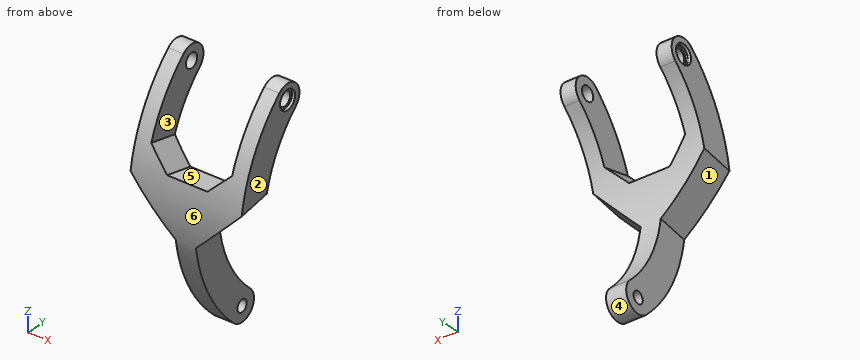
from build123d import *

# Parameters (mm, degrees)
SKETCH_1_R               = 1.175
SKETCH_1_R_2             = 1.425
EXTRUDE_1_DEPTH          = 11
CUT_EXTRUDE_1_DEPTH      = 8
CUT_EXTRUDE_1_DEPTH_BACK = 8
SKETCH_1_6_R             = 1.425
SKETCH_4_R               = 1.175
CUT_EXTRUDE_3_DEPTH      = 9
CUT_EXTRUDE_START        = -0.6
SKETCH_6_R               = 1.9
CUT_EXTRUDE_5_DEPTH      = 35.929603411
SKETCH_3_R               = 1.85
CUT_EXTRUDE_2_DEPTH      = 1
CHAMFER_2_SIZE           = 10
CHAMFER_3_SIZE           = 4


with BuildPart() as part:
    # 草图1 → 凸台-拉伸1 (new, symmetric)
    with BuildSketch(Plane(origin=(0, 0, 0), x_dir=(0, 0, -1), z_dir=(1, 0, 0))):
        with BuildLine():
            ThreePointArc((-22.696428571, -2.043453335), (0, -11.927768877), (22.696428571, -2.043453335))
            ThreePointArc((22.696428571, -2.043453335), (22.543453335, 2.196428571), (18.303571429, 2.043453335))
            ThreePointArc((18.303571429, 2.043453335), (0, -5.927768877), (-18.303571429, 2.043453335))
            ThreePointArc((-18.303571429, 2.043453335), (-22.543453335, 2.196428571), (-22.696428571, -2.043453335))
        make_face()
        with Locations((20.5, 0)):
            Circle(SKETCH_1_R, mode=Mode.SUBTRACT)
        with Locations((-20.5, 0)):
            Circle(SKETCH_1_R_2, mode=Mode.SUBTRACT)
    extrude(amount=EXTRUDE_1_DEPTH, both=True)

    # 草图1<6> → 切除-拉伸1 (cut, two sides: drawn at the far end of the back side and taken through both)
    with BuildSketch(Plane(origin=(0, 0, 0), x_dir=(0, 0, -1), z_dir=(1, 0, 0)).offset(-CUT_EXTRUDE_1_DEPTH_BACK)):
        with BuildLine():
            ThreePointArc((-22.696428571, -2.043453335), (-15.296359873, -7.89110277), (-6.48036682, -11.242861585))
            Line((-6.48036682, -11.242861585), (-5.226102274, -5.375424287))
            ThreePointArc((-5.226102274, -5.375424287), (-12.335774091, -2.672392985), (-18.303571429, 2.043453335))
            ThreePointArc((-18.303571429, 2.043453335), (-22.543453335, 2.196428571), (-22.696428571, -2.043453335))
        make_face()
        with Locations((-20.5, 0)):
            Circle(SKETCH_1_6_R, mode=Mode.SUBTRACT)
    extrude(amount=CUT_EXTRUDE_1_DEPTH + CUT_EXTRUDE_1_DEPTH_BACK, mode=Mode.SUBTRACT)

    # 草图4 → 切除-拉伸3 (cut)
    with BuildSketch(Plane(origin=(11, 0, 0), x_dir=(0, 0, -1), z_dir=(1, 0, 0))):
        with BuildLine():
            ThreePointArc((18.303571429, 2.043453335), (11.941686142, -2.891287085), (4.341204442, -5.547962703))
            Line((4.341204442, -5.547962703), (5.383093508, -11.456809221))
            ThreePointArc((5.383093508, -11.456809221), (14.807690816, -8.162531455), (22.696428571, -2.043453335))
            ThreePointArc((22.696428571, -2.043453335), (23.487928503, 0.268855462), (22.296358841, 2.402726558))
            ThreePointArc((22.296358841, 2.402726558), (20.231144538, 2.987928503), (18.303571429, 2.043453335))
        make_face()
        with Locations((20.5, 0)):
            Circle(SKETCH_4_R, mode=Mode.SUBTRACT)
    cut_extrude_3 = extrude(amount=-CUT_EXTRUDE_3_DEPTH, mode=Mode.SUBTRACT)

    # 草图6 → 切除-拉伸5 (cut)
    with BuildSketch(Plane(origin=(11, 0, 0), x_dir=(0, 0, -1), z_dir=(1, 0, 0)).offset(CUT_EXTRUDE_START)):
        with Locations(Location((-20.5, 0, 0), (0, 0, 180))):
            Circle(SKETCH_6_R)
    cut_extrude_5 = extrude(amount=CUT_EXTRUDE_5_DEPTH, mode=Mode.SUBTRACT)

    # 镜向3: 切除-拉伸3, 切除-拉伸5 across plane
    add(cut_extrude_3.mirror(Plane(origin=(0, 0, 0), x_dir=(0, 0, 1), z_dir=(1, 0, 0))), mode=Mode.SUBTRACT)
    add(cut_extrude_5.mirror(Plane(origin=(0, 0, 0), x_dir=(0, 0, 1), z_dir=(1, 0, 0))), mode=Mode.SUBTRACT)

    # 草图3 → 切除-拉伸2 (cut)
    with BuildSketch(Plane.ZY.offset(11)):
        with Locations((20.5, 0)):
            Circle(SKETCH_3_R)
    extrude(amount=-CUT_EXTRUDE_2_DEPTH, mode=Mode.SUBTRACT)

    # 倒角2
    # the kernel refuses this chamfer: 10 mm, written as the material it adds along each edge
    # the kernel refuses this chamfer: 10 mm, written as the material it takes off along each edge
    with BuildSketch(Plane(origin=(-11, 19.778170746, 0.124476202), x_dir=(-0.027495876610586313, -0.1735825242275637, 0.9844354138551714), z_dir=(0, -0.9848077530122094, -0.17364817766692373))) as chamfer_2_2_piece_1_section:
        Polygon((CHAMFER_2_SIZE * 0.999621916911, -CHAMFER_2_SIZE * 0.0274958766106), (-CHAMFER_2_SIZE * 0.0274958766106, -CHAMFER_2_SIZE * 0.999621916911), (0, 0), align=None)
    chamfer_2_2_piece_1 = extrude(amount=57.433659759, mode=Mode.PRIVATE)
    chamfer_2_2_piece_1 = split(chamfer_2_2_piece_1, bisect_by=Plane(origin=(-2, -8.783186583, -1.465639678), z_dir=(-1, 0, 0)), keep=Keep.TOP, mode=Mode.PRIVATE)
    add(chamfer_2_2_piece_1, mode=Mode.SUBTRACT)
    with BuildSketch(Plane(origin=(11, 19.778170746, 0.124476202), x_dir=(-0.9996219169112968, 0.004774608866782908, -0.027078152461972493), z_dir=(0, -0.9848077530122094, -0.17364817766692373))) as chamfer_2_2_piece_2_section:
        Polygon((CHAMFER_2_SIZE * 0.999621916911, -CHAMFER_2_SIZE * 0.0274958766106), (-CHAMFER_2_SIZE * 0.0274958766106, -CHAMFER_2_SIZE * 0.999621916911), (0, 0), align=None)
    chamfer_2_2_piece_2 = extrude(amount=57.433659759, mode=Mode.PRIVATE)
    chamfer_2_2_piece_2 = split(chamfer_2_2_piece_2, bisect_by=Plane(origin=(2, -8.783186583, -1.465639678), z_dir=(1, 0, 0)), keep=Keep.TOP, mode=Mode.PRIVATE)
    add(chamfer_2_2_piece_2, mode=Mode.SUBTRACT)

    # 倒角3
    chamfer_3_edges = [part.edges().sort_by_distance(p)[0] for p in [
        (8, -8.309142936, 5.853234547),
        (-8, -8.309142936, 5.853234547),
    ]]
    chamfer(chamfer_3_edges, length=CHAMFER_3_SIZE)


solid = part.part
Build history of the part. All positions in model axes, mm. Face numbers are marked on the shaded views. A direction names the side the tool comes from. Give positions to 0.01 mm unless a question says otherwise; leave off trailing zeros. Write each loop counter-clockwise with the first axis right and the second up, starting at its lowest first coordinate (ties: lowest second). Pieces come first, ordered by that corner, then holes. Notation, with made-up numbers: (3, 21) - (60, 21) arc R23 ccw to (60, 50) - close; hole circle Ø11 at (6, 82.25). An arc over 180 degrees is marked (long way). Use one line per item in the form item = value. Start each with the question number.
1. Band-saw the part on D-D on z = 20.5. Write the cut outline in (x, y) (3 decimals).
2. Two-plate mould, pull along X, no slides. Class the marked faces 1, 2, 3 and 4: released by +X, released by -X, zero draft, split by the parting line, or undercut.
3. Band-saw the part on B-B on z = 7.5. Write the cut outline in (x, y), plus the area to 3 significant figures.
4. Band-saw the part on A-A on x = -0.25. Write the cut outline in (y, z) (3 decimals), plus the area to 3 significant figures.
5. 3-axis set-ups, long thin cutter, end or side, ignore diameter. For the marked faces 5 and 6: which of +Z, -Z, +X, -X, +Y, -Y reach the whole face in a straight line?
6. Probe line 1 (X direction, y = -3.25, z = 16); line 2 (Y direction, x = -0.35, z = -20.5) (3 decimals); line 3 (Z direction, x = 0.25, y = 0.75). List the from-to ranges inside material, lowest first. Write a range as [from, to].
7. Drop flat-ended pins along their axis: pin 1 Ø1 at (x, y) = (-8, -4.5) entering from +Z; pin 2 Ø2 at (x, z) = (-2.5, -13.5) entering from +Y; pin 3 Ø1.1 at (y, z) = (1, 21) entering from -X. Give the stop position or say it passes through.
8. Band-saw the part on C-C on y = -2.5. Write the cut outline in (x, z), plus the area to 3 significant figures.
Conclusion:
q1.outline = (-11, -4.182) - (-8, -4.182) - (-8, -1.425) - (-10, -1.425) - (-10, -1.85) - (-10.4, -1.85) - (-10.4, -1.9) - (-11, -1.9) - close; (-11, 1.9) - (-10.4, 1.9) - (-10.4, 1.85) - (-10, 1.85) - (-10, 1.425) - (-8, 1.425) - (-8, 3) - (-11, 3) - close; (8, -4.182) - (11, -4.182) - (11, -1.9) - (10.4, -1.9) - (10.4, -1.425) - (8, -1.425) - close; (8, 1.425) - (10.4, 1.425) - (10.4, 1.9) - (11, 1.9) - (11, 3) - (8, 3) - close
q2.face_1 = released by -X
q2.face_2 = released by +X
q2.face_3 = undercut
q2.face_4 = zero draft
q3.outline = (-11, -11.01) - (-5.05, -11.01) - (-6.35, -4.78) - (-11, -4.78) - close; (5.05, -11.01) - (11, -11.01) - (11, -4.78) - (6.35, -4.78) - close
q3.area = 66.1 mm²
q4.outline = (-11.243, 6.48) arc R31 ccw to (-2.043, -22.696) arc R3 ccw to (2.043, -18.304) arc R25 cw to (-5.375, 5.226) - close; hole circle Ø2.35 at (0, -20.5)
q4.area = 183 mm²
q5.face_5 = +Z, +Y
q5.face_6 = +X, -X, -Y
q6.line_1 = [-11, -8], [8, 11]
q6.line_2 = [-4.182, -1.175], [1.175, 3]
q6.line_3 = [-23.4, -21.4], [-19.6, -17.01]
q7.pin_1 = 20.7
q7.pin_2 = -1.39
q7.pin_3 = -10
q8.outline = (-11, 12.63) - (-8, 12.63) - (-8, 22.26) - (-11, 22.26) - close; (-2, -22.26) - (2, -22.26) - (2, -12.63) - (-2, -12.63) - close; (8, 12.63) - (11, 12.63) - (11, 22.26) - (8, 22.26) - close
q8.area = 96.3 mm²
